from build123d import *

# Parameters (mm, degrees)
SKETCH1_R               = 18.5
BOSS_EXTRUDE1_DEPTH     = 22.5
SKETCH2_R               = 1.6
CUT_EXTRUDE1_DEPTH      = 3.5
BOSS_EXTRUDE2_DEPTH     = 36.3
BOSS_EXTRUDE3_DEPTH     = 6.3
SKETCH4_R               = 14.5
BOSS_EXTRUDE4_DEPTH     = 37.8
SKETCH5_R               = 5
BOSS_EXTRUDE5_DEPTH     = 3
SKETCH6_R               = 1
BOSS_EXTRUDE6_DEPTH     = 9
SKETCH7_W               = 0.5
SKETCH7_H               = 3
BOSS_EXTRUDE7_DEPTH     = 6.5
CUT_EXTRUDE2_DEPTH      = 0.5
FILLET1_R               = 0.5
CUT_EXTRUDE3_DEPTH      = 67.7078706
CUT_EXTRUDE3_DEPTH_BACK = 67.7078706
SKETCH9_R               = 1.6


with BuildPart() as part:
    # Sketch1 → Boss-Extrude1 (new body)
    with BuildSketch(Plane.XY):
        with Locations(Location((0, 0, 0), (0, 0, 180))):
            Circle(SKETCH1_R)
    extrude(amount=BOSS_EXTRUDE1_DEPTH)

    # Sketch2 → Cut-Extrude1 (cut)
    with BuildSketch(Plane.XY.offset(22.5)):
        with Locations((-7.75, 13.423393759)):
            Circle(SKETCH2_R)
        with Locations((7.75, 13.423393759)):
            Circle(SKETCH2_R)
        with Locations((-15.5, 0)):
            Circle(SKETCH2_R)
        with Locations((-7.75, -13.423393759)):
            Circle(SKETCH2_R)
        with Locations((7.75, -13.423393759)):
            Circle(SKETCH2_R)
        with Locations((15.5, 0)):
            Circle(SKETCH2_R)
    extrude(amount=-CUT_EXTRUDE1_DEPTH, mode=Mode.SUBTRACT)

    # Sketch3 → Boss-Extrude2 (add)
    with BuildSketch(Plane.XY.offset(22.5)):
        with BuildLine():
            ThreePointArc((0, 10), (-3, 7), (0, 4))
            Line((0, 4), (0, 10))
        make_face()
        with BuildLine():
            Line((0, 10), (0, 4))
            ThreePointArc((0, 4), (2.121320344, 4.878679656), (3, 7))
            ThreePointArc((3, 7), (2.121320344, 9.121320344), (0, 10))
        make_face()
    extrude(amount=BOSS_EXTRUDE2_DEPTH)

    # Sketch3_3 → Boss-Extrude3 (add)
    with BuildSketch(Plane.XY.offset(22.5)):
        with BuildLine():
            ThreePointArc((0, 13), (-6, 7), (0, 1))
            Line((0, 1), (0, 4))
            ThreePointArc((0, 4), (-3, 7), (0, 10))
            Line((0, 10), (0, 13))
        make_face()
        with BuildLine():
            Line((0, 4), (0, 1))
            ThreePointArc((0, 1), (4.242640687, 2.757359313), (6, 7))
            ThreePointArc((6, 7), (4.242640687, 11.242640687), (0, 13))
            Line((0, 13), (0, 10))
            ThreePointArc((0, 10), (2.121320344, 9.121320344), (3, 7))
            ThreePointArc((3, 7), (2.121320344, 4.878679656), (0, 4))
        make_face()
    extrude(amount=BOSS_EXTRUDE3_DEPTH)

    # Sketch4 → Boss-Extrude4 (add)
    with BuildSketch(Plane(origin=(0, 0, 0), x_dir=(-1, 0, 0), z_dir=(0, 0, -1))):
        with Locations(Location((0, 0, 0), (0, 0, 180))):
            Circle(SKETCH4_R)
    extrude(amount=BOSS_EXTRUDE4_DEPTH)

    # Sketch5 → Boss-Extrude5 (add)
    with BuildSketch(Plane(origin=(0, 0, -37.8), x_dir=(-1, 0, 0), z_dir=(0, 0, -1))):
        Circle(SKETCH5_R)
    extrude(amount=BOSS_EXTRUDE5_DEPTH)

    # Sketch6 → Boss-Extrude6 (add)
    with BuildSketch(Plane(origin=(0, 0, -40.8), x_dir=(-1, 0, 0), z_dir=(0, 0, -1))):
        Circle(SKETCH6_R)
    extrude(amount=BOSS_EXTRUDE6_DEPTH)

    # Sketch7 → Boss-Extrude7 (add)
    with BuildSketch(Plane(origin=(0, 0, -37.8), x_dir=(-1, 0, 0), z_dir=(0, 0, -1))):
        with Locations((-11.75, 0)):
            Rectangle(SKETCH7_W, SKETCH7_H)
        with Locations((11.75, 0)):
            Rectangle(SKETCH7_W, SKETCH7_H)
    extrude(amount=BOSS_EXTRUDE7_DEPTH)

    # Sketch8 → Cut-Extrude2 (cut)
    with BuildSketch(Plane(origin=(12, 0, 0), x_dir=(0, 0, -1), z_dir=(1, 0, 0))):
        with BuildLine():
            Line((42.865122037, -0.320114275), (41.665122037, -0.320114275))
            ThreePointArc((41.665122037, -0.320114275), (41.345007763, 0), (41.665122037, 0.320114275))
            Line((41.665122037, 0.320114275), (42.865122037, 0.320114275))
            ThreePointArc((42.865122037, 0.320114275), (43.185236312, 0), (42.865122037, -0.320114275))
        make_face()
    cut_extrude2 = extrude(amount=-CUT_EXTRUDE2_DEPTH, mode=Mode.SUBTRACT)

    # Mirror2: Cut-Extrude2 across plane
    add(cut_extrude2.mirror(Plane(origin=(0, 0, 0), x_dir=(0, 0, 1), z_dir=(1, 0, 0))), mode=Mode.SUBTRACT)

    # Fillet1
    fillet1_edges = [part.edges().sort_by_distance(p)[0] for p in [
        (11.75, -1.5, -44.3),
        (11.75, 1.5, -44.3),
        (-11.75, 1.5, -44.3),
        (-11.75, -1.5, -44.3),
    ]]
    fillet(fillet1_edges, radius=FILLET1_R)

    # Chamfer1: read off the stored shape, not the designer's step
    # Chamfer1 outline → Chamfer1 (revolve, cut)
    with BuildSketch(Plane.XZ):
        Polygon((18.5, 22.5), (18.3, 22.5), (18.5, 22.3), align=None)
    revolve(axis=Axis((0, 0, 0), (0, 0, 1)), mode=Mode.SUBTRACT)

    # Chamfer1 2 outline → Chamfer1 2 (revolve, cut)
    with BuildSketch(Plane.XZ.offset(-7)):
        Polygon((6, 28.8), (5.8, 28.8), (6, 28.6), align=None)
        Polygon((2.8, 58.8), (3, 58.6), (3, 58.8), align=None)
    revolve(axis=Axis((0, 7, 0), (0, 0, 1)), mode=Mode.SUBTRACT)

    # Sketch9 → Cut-Extrude3 (cut, two sides: drawn at the far end of the back side and taken through both)
    with BuildSketch(Plane(origin=(0, 7, 0), x_dir=(1, 0, 0), z_dir=(0, 1, 0)).offset(-CUT_EXTRUDE3_DEPTH_BACK)):
        with Locations(Location((0, -50.8, 0), (0, 0, 270))):
            Circle(SKETCH9_R)
    extrude(amount=CUT_EXTRUDE3_DEPTH + CUT_EXTRUDE3_DEPTH_BACK, mode=Mode.SUBTRACT)


solid = part.part
Verification items for the finished model (mm, model axes). A direction names the side the tool comes from. Give positions to 0.01 mm unless a question says otherwise; leave off trailing zeros. Write each loop counter-clockwise with the first axis right and the second up, starting at its lowest first coordinate (ties: lowest second). Pieces come first, ordered by that corner, then holes. Notation, with made-up numbers: M -13,-17 L 43,-17 A13 cw 43,6 Z; hole C -28.75,59.5 d6. An arc over 180 degrees is marked long. Write item = value, one per line.
(1) Sectioned sample at B-B (z = 21). Record the cut outline in (x, y).
Found:
outline = C 0,0 d37; hole C -15.5,0 d3.2; hole C -7.75,-13.42 d3.2; hole C -7.75,13.42 d3.2; hole C 7.75,-13.42 d3.2; hole C 7.75,13.42 d3.2; hole C 15.5,0 d3.2
(2) Access from +Z, -Z, +X, -X, +Y, -Y to the whole of each face (thin tool, end or side, straight path). Record for faces 1 (the face through (-16, 0, 19)), 2 (the face through (12, 0, -41)), 3 (the face through (-12, 0, -41)), 4 (the face through (0, -1, -45)), 5 (the face through (-11.5, 0, -41)).
Found:
face_1 = +Z
face_2 = -Z, +X, +Y, -Y
face_3 = -Z, -X, +Y, -Y
face_4 = -Z
face_5 = -Z, +Y, -Y
(3) Go/stop test with flat-tipped pins: pin 1 Ø3.5 at (y, z) = (0, -42.5) entering from +X; pin 2 Ø2 at (y, z) = (-1.5, -27) entering from +X; pin 3 Ø0.6 at (x, z) = (-12, -42) entering from +Y. Record where each tip stops, or that it passes through.
Found:
pin_1 = 12
pin_2 = 14.49
pin_3 = 1.5
(4) Draft check along Y on faces 6 (the face through (11, 10, 0)), 7 (the face through (6.691, 12.864, -18.635)), 8 (the face through (-8.097, -14.985, 20.774)). Enter one of: released by +Y, released by -Y, zero draft, split by the parting line, or undercut.
Found:
face_6 = zero draft
face_7 = split by the parting line
face_8 = undercut
(5) Sectioned sample at A-A (z = 50.8). Record the cut outline in (x, y), then the cut area to 3 significant figures.
Found:
outline = M -1.6,4.46 L -1.6,9.54 A3 ccw Z; M 1.6,4.46 A3 ccw 1.6,9.54 Z
area = 10.0 mm2
(6) Material ranges on line 1 (Y direction, x = 7, z = 20); line 2 (Z direction, x = 14, y = -9); line 3 (Z direction, x = -5.5, y = 9.5), recorded low to high.
Found:
line_1 = -17.12 to -14.84, -12.01 to 12.01, 14.84 to 17.12
line_2 = 0 to 22.5
line_3 = -37.8 to 22.5
(7) Sectioned sample at C-C (z = -2). Record the cut outline in (x, y), then the cut area to 3 significant figures.
Found:
outline = C 0,0 d29
area = 661 mm2
